Here's how the part is built. I have some questions about the finished solid (model axes, mm). Coordinates: 2 decimals unless noted, no trailing zeros. Loops run counter-clockwise (first coordinate to the right, second up) from the corner with the lowest first, then second, coordinate; pieces in that order, holes last. Notation, with made-up numbers: M 28.25,25 L 66.25,25 A23 ccw 66.25,64 Z; hole C -19.75,80 d5. An arc over 180 degrees is marked long. Use CSV: the item, a comma, the result in double quotes. Start each with the question number.
Q1. If we section it at B-B (y = 10): Please give me the cut outline in (x, z), and give its area (3 significant figures).
Q2. If we section it at A-A (x = 170): Please give me the cut outline in (y, z).
Q3. Please list where these lines run through material, in increasing order: probe 1 along X at (y, z) = (95, 0.5); probe 2 along Y at (x, z) = (10, 0.9); probe 3 along Y at (x, z) = (11.5, 1.3). Write a range as [from, to].
Q4. For pin 1 Ø6.5 at (x, y) = (170, 10) entering from +Z, with a flat end and sliding along its axis, tell me the tip position at first contact or that it passes through.
from build123d import *

# Parameters (mm, degrees)
EXTRUDE_1_DEPTH          = 1.6
CUT_EXTRUDE_1_DEPTH      = 209.392802179
CUT_EXTRUDE_1_DEPTH_BACK = 209.392802179
SKETCH_2_R               = 4


with BuildPart() as part:
    # ｽｹｯﾁ1 → ﾎﾞｽ - 押し出し1 (new body)
    with BuildSketch(Plane.XY):
        with BuildLine():
            Line((5, 0), (175, 0))
            ThreePointArc((175, 0), (178.535533906, 1.464466094), (180, 5))
            Line((180, 5), (180, 100))
            ThreePointArc((180, 100), (178.535533906, 103.535533906), (175, 105))
            Line((175, 105), (5, 105))
            ThreePointArc((5, 105), (1.464466094, 103.535533906), (0, 100))
            Line((0, 100), (0, 5))
            ThreePointArc((0, 5), (1.464466094, 1.464466094), (5, 0))
        make_face()
    extrude(amount=EXTRUDE_1_DEPTH)

    # ｽｹｯﾁ2 → ｶｯﾄ - 押し出し1 (cut, two sides: drawn at the far end of the back side and taken through both)
    with BuildSketch(Plane.XY.offset(-CUT_EXTRUDE_1_DEPTH_BACK)):
        with Locations((10, 10)):
            Circle(SKETCH_2_R)
        with Locations((10, 95)):
            Circle(SKETCH_2_R)
        with Locations((170, 10)):
            Circle(SKETCH_2_R)
        with Locations((170, 95)):
            Circle(SKETCH_2_R)
    extrude(amount=CUT_EXTRUDE_1_DEPTH + CUT_EXTRUDE_1_DEPTH_BACK, mode=Mode.SUBTRACT)


solid = part.part
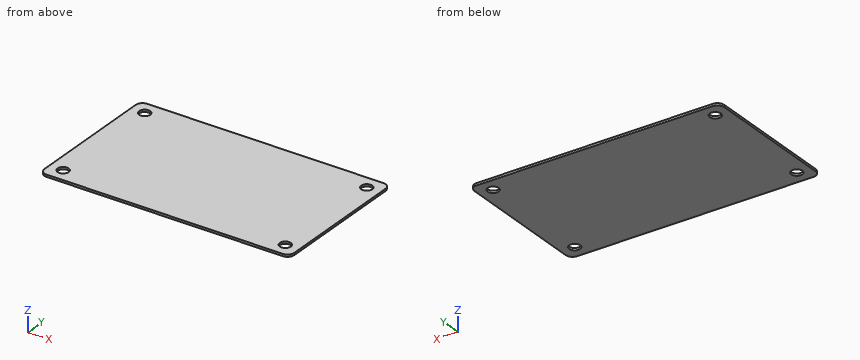
Results below:
1,outline,"M 0,0 L 6,0 L 6,1.6 L 0,1.6 Z; M 14,0 L 166,0 L 166,1.6 L 14,1.6 Z; M 174,0 L 180,0 L 180,1.6 L 174,1.6 Z"
1,area,"262 mm^2"
2,outline,"M 0,0 L 6,0 L 6,1.6 L 0,1.6 Z; M 14,0 L 91,0 L 91,1.6 L 14,1.6 Z; M 99,0 L 105,0 L 105,1.6 L 99,1.6 Z"
3,probe 1,"[0, 6], [14, 166], [174, 180]"
3,probe 2,"[0, 6], [14, 91], [99, 105]"
3,probe 3,"[0, 6.29], [13.71, 91.29], [98.71, 105]"
4,pin 1,"through"
